Autodesk Inventor part; units mm, degrees
ref_plane "YZ Plane" through (0, 0, 0) normal (1, 0, 0) x (0, 1, 0)
ref_plane "XZ Plane" through (0, 0, 0) normal (0, 1, 0) x (-1, 0, 0)
ref_plane "XY Plane" through (0, 0, 0) normal (0, 0, 1) x (1, 0, 0)
sketch "Sketch1" plane through (0, 0, 0) normal (0, 1, 0) x (-1, 0, 0)
  line L0 (25.4, 0) -> (-25.4, 0) construction
  line L1 (25.4, 25.4) -> (-25.4, 25.4)
  line L2 (-25.4, -25.4) -> (25.4, -25.4)
  arc A0 (25.4, -25.4) -> (25.4, 25.4) centre (25.4, 0) ccw
  arc A1 (-25.4, 25.4) -> (-25.4, -25.4) centre (-25.4, 0) ccw
  point P0 (0, 0)
  dimension "d0" = 50.8
  dimension "d1" = 25.4
extrude "Extrusion1" add sketch "Sketch1" along normal blind 6.35
sketch "Sketch2" plane through (0, 6.35, 0) normal (0, 1, 0) x (1, 0, 0)
  line L0 (25.4, 0) -> (-25.4, 0) construction
  line L1 (25.4, 19.05) -> (-25.4, 19.05)
  line L2 (-25.4, -19.05) -> (25.4, -19.05)
  arc A0 (25.4, -19.05) -> (25.4, 19.05) centre (25.4, 0) ccw
  arc A1 (-25.4, 19.05) -> (-25.4, -19.05) centre (-25.4, 0) ccw
  line L3 (25.4, 25.4) -> (-25.4, 25.4)
  line L4 (12.7, -19.05) -> (12.7, -12.7)
  line L5 (12.7, -12.7) -> (39.599, -12.7)
  line L6 (12.7, 19.05) -> (12.7, 12.7)
  line L7 (12.7, 12.7) -> (39.599, 12.7)
  circle A2 centre (-25.4, 0) radius 12.7
  point P0 (0, 0)
  point P1 (0, 0)
  point P2 (12.7, -15.875)
  point P3 (39.599, 12.7)
  dimension "d4" = 19.05
  dimension "d5" = 38.1
  dimension "d6" = 25.4
  dimension "d7" = 25.4
extrude "Extrusion2" add sketch "Sketch2" along normal blind 12.7 contours L6 L7 A0 L5 L4 L2 A1 L1
sketch "Sketch3" plane through (0, 19.05, 0) normal (0, 1, 0) x (1, 0, 0)
  arc A0 (25.4, -25.4) -> (25.4, 25.4) centre (25.4, 0) ccw
  circle A1 centre (25.4, 0) radius 6.35
  point P0 (0, 0)
  dimension "d10" = 12.7
extrude "Extrusion3" add sketch "Sketch3" along normal blind 6.35
properties part number "PivotLock"
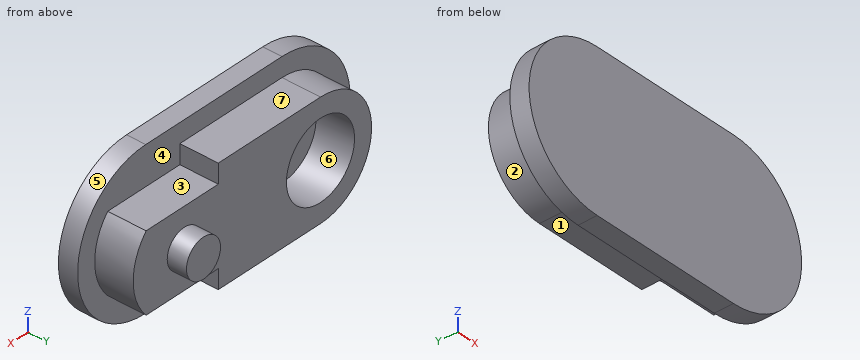
The model under review builds one solid part; all positions refer to its coordinate system, in mm. Face numbers are marked on the shaded views. A direction names the side the tool comes from. Coordinates: 2 decimals unless noted, no trailing zeros. Loops run counter-clockwise (first coordinate to the right, second up) from the corner with the lowest first, then second, coordinate; pieces in that order, holes last.
(1) Consider section D-D, the plane y = 3. Give the boundary of the cut face in (x, z).
Determined:
outline: (-25.4, -25.4) - (25.4, -25.4) arc R25.4 ccw to (25.4, 25.4) - (-25.4, 25.4) arc R25.4 ccw to start
(2) Consider section C-C, the plane z = 0. Give the boundary of the cut face in (x, y).
Determined:
outline: (-50.8, 0) - (50.8, 0) - (50.8, 6.35) - (44.45, 6.35) - (44.45, 19.05) - (31.75, 19.05) - (31.75, 25.4) - (19.05, 25.4) - (19.05, 19.05) - (-12.7, 19.05) - (-12.7, 6.35) - (-38.1, 6.35) - (-38.1, 19.05) - (-44.45, 19.05) - (-44.45, 6.35) - (-50.8, 6.35) - close
(3) Tool access review of the marked faces 1, 2, 3 and 4: name each direction out of +Z, -Z, +X, -X, +Y, -Y from which nothing blocks a thin tool from reaching the whole face with its end or side.
Determined:
face 1: -Z, +X, -X, +Y
face 2: -X, +Y
face 3: +Z, +X, +Y
face 4: +Y
(4) Consider section B-B, the plane x = 0. Give the boundary of the cut face in (y, z).
Determined:
outline: (0, -25.4) - (6.35, -25.4) - (6.35, -19.05) - (19.05, -19.05) - (19.05, 19.05) - (6.35, 19.05) - (6.35, 25.4) - (0, 25.4) - close
(5) Consider section A-A, the plane y = 16. Give the boundary of the cut face in (x, z).
Determined:
outline: (-25.4, -19.05) - (12.7, -19.05) - (12.7, -12.7) - (39.6, -12.7) arc R19.05 ccw to (39.6, 12.7) - (12.7, 12.7) - (12.7, 19.05) - (-25.4, 19.05) arc R19.05 ccw to start; hole circle Ø25.4 at (-25.4, 0)
(6) Insertion check: P1, Ø8, axis at y = 11, z = 1.5, coming from the -X side; P2, Ø3, axis at y = 11.5, z = -17, coming from the +X side; P3, Ø14, axis at x = -11.5, y = 9.5, coming from the +Z side; P4, Ø19, axis at x = -10.5, z = -1.5, coming from the +Y side. Each pin has a flat end and moves straight along its axis. Give the tip position at first contact, or say it passes through.
Determined:
P1: stops at x = -44.45
P2: stops at x = 12.7
P3: stops at z = 25.4
P4: stops at y = 19.05
(7) Draft analysis for pull direction X (two halves, no side actions). For the marked faces 5, 6 and 7, state which applies: +X half, -X half, draft (parallel to the pull), parting line (faces both ways), or undercut.
Determined:
face 5: +X half
face 6: undercut
face 7: draft
(8) Wall thickness on L1, parallel to Z at x = -25.4, y = 12; L2, parallel to X at y = 13.25, z = 0; L3, parallel to Y at x = -21.5, z = 0: over which ranges is each line inside the solid? List them lowest first.
Determined:
L1: z = -19.05 to -12.7, 12.7 to 19.05
L2: x = -44.45 to -38.1, -12.7 to 44.45
L3: y = 0 to 6.35
